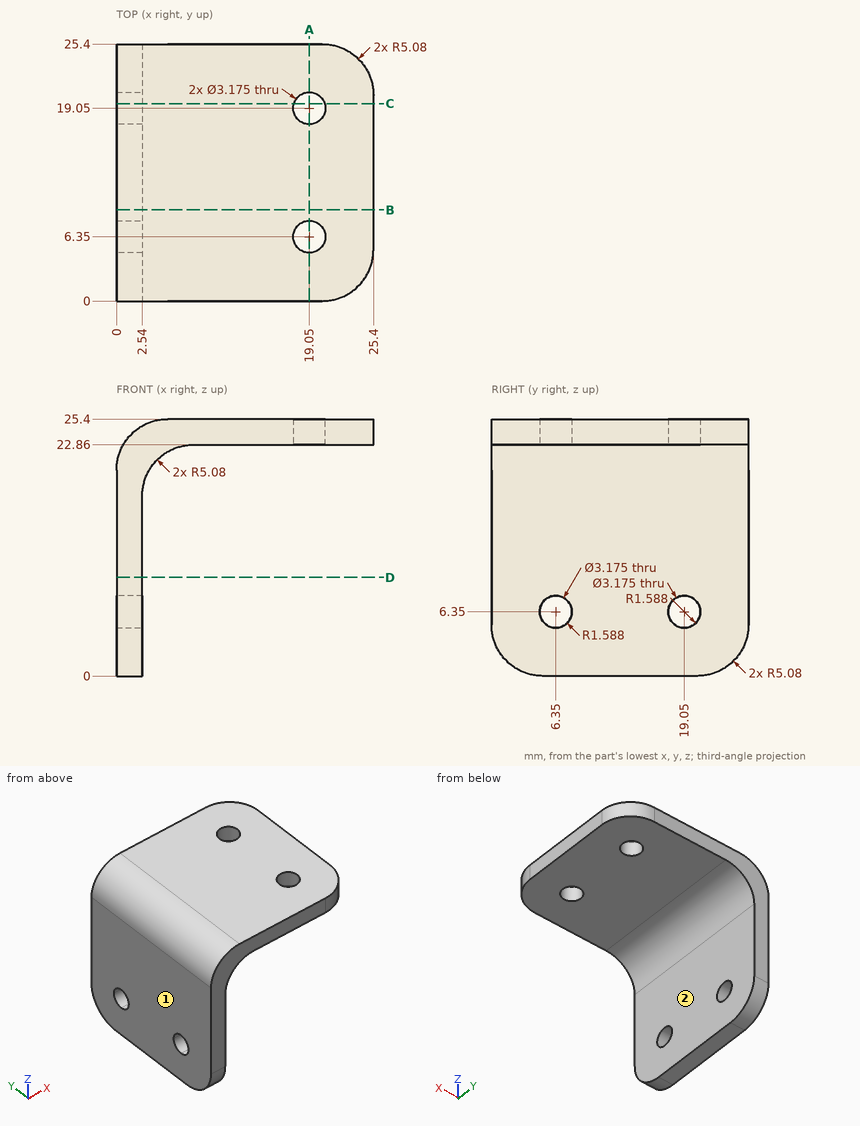
Could you check a few things on this drawing? It's one solid part, dimensions in mm from its lowest x, y, z. A direction names the side the tool comes from. Coordinates: 2 decimals unless noted, no trailing zeros. Loops run counter-clockwise (first coordinate to the right, second up) from the corner with the lowest first, then second, coordinate; pieces in that order, holes last. Notation, with made-up numbers: (4, 67) - (24, 67) arc R21 ccw to (24, 87) - close; hole circle Ø6 at (-4.5, 30.25). An arc over 180 degrees is marked (long way). Return JSON: item names as keys, results as strings. Group by question number.
Item 1: Will these pins go through, and if not, where does the flat tip stop? P1, Ø1.9, axis at x = 19.05, y = 6.35, coming from the +Z side; P2, Ø12, axis at x = 9.5, z = 17, coming from the -Y side; P3, Ø2, axis at y = 6, z = 19.5, coming from the +X side; P4, Ø3.5, axis at y = 19.05, z = 6.35, coming from the +X side.
Item 2: If we section it at B-B on y = 9: Write out the boundary of the cut face in (x, z).
Item 3: If we section it at C-C on y = 19.5: Write out the boundary of the cut face in (x, z), and give its area (3 significant figures).
Item 4: On a 3-axis mill with a long thin cutter (end or side, diameter ignored), from which of +Z, -Z, +X, -X, +Y, -Y can I reach the whole of each face in a straight line? I mean the marked faces 1 and 2. Say none if no direction works.
Item 5: I need wall thicknesses on line 1 (Y direction, x = 19.05, z = 24.5); line 2 (Z direction, x = 13.25, y = 6.5); line 3 (X direction, y = 5.25, z = 12.5). Which ranges of each line are inside material? Lowest first, please. Write a range as from..to.
Item 6: If we section it at D-D on z = 9.75: Write out the boundary of the cut face in (x, y).
Item 7: If we section it at A-A on x = 19.05: Write out the boundary of the cut face in (y, z).
Calculated:
{
 "1": {"P1": "passes through", "P2": "stops at y = 0", "P3": "stops at x = 3.33", "P4": "stops at x = 2.54"},
 "2": {"outline": "(0, 0) - (2.54, 0) - (2.54, 17.78) arc R5.08 cw to (7.62, 22.86) - (25.4, 22.86) - (25.4, 25.4) - (5.08, 25.4) arc R5.08 ccw to (0, 20.32) - close"},
 "3": {"outline": "(0, 0) - (2.54, 0) - (2.54, 4.83) - (0, 4.83) - close; (0, 7.87) - (2.54, 7.87) - (2.54, 17.78) arc R5.08 cw to (7.62, 22.86) - (17.53, 22.86) - (17.53, 25.4) - (5.08, 25.4) arc R5.08 ccw to (0, 20.32) - close; (20.57, 22.86) - (25.4, 22.86) - (25.4, 25.4) - (20.57, 25.4) - close", "area": "107 mm^2"},
 "4": {"face 1": "+Z, -Z, -X, +Y, -Y", "face 2": "-Z, +X, +Y, -Y"},
 "5": {"line 1": "y = 0..4.76, 7.94..17.46, 20.64..25.4", "line 2": "z = 22.86..25.4", "line 3": "x = 0..2.54"},
 "6": {"outline": "(0, 0) - (2.54, 0) - (2.54, 25.4) - (0, 25.4) - close"},
 "7": {"outline": "(0, 22.86) - (4.76, 22.86) - (4.76, 25.4) - (0, 25.4) - close; (7.94, 22.86) - (17.46, 22.86) - (17.46, 25.4) - (7.94, 25.4) - close; (20.64, 22.86) - (25.4, 22.86) - (25.4, 25.4) - (20.64, 25.4) - close"}
}
